Source: CAD feature listing. Evaluate the final solid. Frame: model axes, mm. Round coordinates to 2 decimals unless told otherwise and drop trailing zeros. Order: outer loops, then holes, each group sorted by start corner. A loop starts at its lowest first (then second) coordinate and runs counter-clockwise, first axis right, second up.
```python
from build123d import *

# Parameters (mm, degrees)
SKETCH1_R           = 29
BOSS_EXTRUDE1_DEPTH = 3
CUT_EXTRUDE1_DEPTH  = 3
SKETCH6_R           = 0.9
BOSS_EXTRUDE3_DEPTH = 2.5
SKETCH7_R           = 0.9
BOSS_EXTRUDE4_DEPTH = 2.5
SKETCH8_R           = 5
CUT_EXTRUDE2_DEPTH  = 3


with BuildPart() as part:
    # Sketch1 → Boss-Extrude1 (new body)
    with BuildSketch(Plane(origin=(0, 0, 0), x_dir=(1, 0, 0), z_dir=(0, 1, 0))):
        with Locations(Location((0, 0, 0), (0, 0, 270))):
            Circle(SKETCH1_R)
    extrude(amount=BOSS_EXTRUDE1_DEPTH)

    # Sketch2 → Cut-Extrude1 (cut)
    with BuildSketch(Plane(origin=(0, 3, 0), x_dir=(1, 0, 0), z_dir=(0, 1, 0))):
        Polygon((0, 29), (6.5, 29), (6.5, 18), (-6.5, 18), (-6.5, 29), align=None)
    extrude(amount=-CUT_EXTRUDE1_DEPTH, mode=Mode.SUBTRACT)

    # Sketch6 → Boss-Extrude3 (add)
    with BuildSketch(Plane(origin=(0, 3, 0), x_dir=(1, 0, 0), z_dir=(0, 1, 0))):
        with Locations(Location((-26, 0, 0), (0, 0, 270))):
            Circle(SKETCH6_R)
        with Locations(Location((26, 0, 0), (0, 0, 270))):
            Circle(SKETCH6_R)
    extrude(amount=BOSS_EXTRUDE3_DEPTH)

    # Sketch7 → Boss-Extrude4 (add)
    with BuildSketch(Plane(origin=(0, 3, 0), x_dir=(1, 0, 0), z_dir=(0, 1, 0))):
        with Locations(Location((0, -26, 0), (0, 0, 270))):
            Circle(SKETCH7_R)
    extrude(amount=BOSS_EXTRUDE4_DEPTH)

    # Sketch8 → Cut-Extrude2 (cut)
    with BuildSketch(Plane(origin=(0, 3, 0), x_dir=(1, 0, 0), z_dir=(0, 1, 0))):
        with Locations(Location((0, 0, 0), (0, 0, 270))):
            Circle(SKETCH8_R)
    extrude(amount=-CUT_EXTRUDE2_DEPTH, mode=Mode.SUBTRACT)


solid = part.part
```
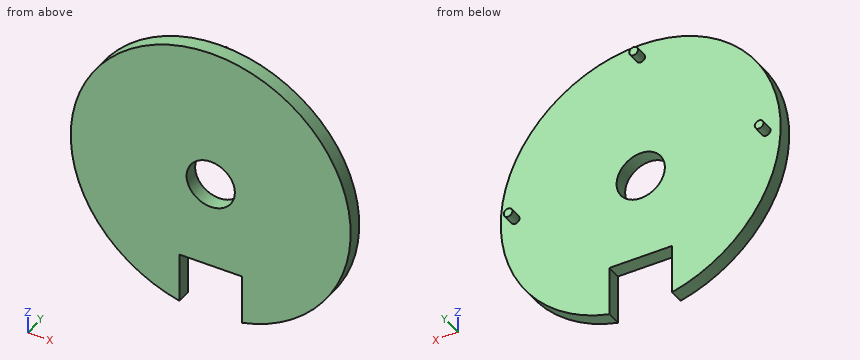
1. Section C-C on y = 1.1. Return loops of the section in (x, z).
2. Section D-D on x = -26. Return loops of the section in (y, z), plus the area to 3 significant figures.
3. Section A-A on x = 0. Return loops of the section in (y, z), plus the area to 4 significant figures.
4. Section B-B on z = 0. Return loops of the section in (x, y), plus the area to 3 significant figures.
5. First-contact query: pin 1 (1 mm diameter, centred on x = -20.5, y = 2.5, fed in from -Z); pin 2 (1.5 mm diameter, centred on x = -3, y = 1, fed in from -Z); pin 3 (4 mm diameter, centred on x = -22.5, z = -0.5, fed in from -Y); pin 4 (2 mm diameter, centred on y = 2, z = 1.5, fed in from -X). Flat tips, straight axial feed; report the tip coordinate or a pass-through.
6. Line query: line 1 along X through (y, z) = (1.1, 0); line 2 along Y through (x, z) = (13.5, -13); line 3 along Z through (x, y) = (-14.5, 1.45). Output: solid intervals per line, ascending.
Result:
1. outline: (-6.5, -28.26) - (-6.5, -18) - (6.5, -18) - (6.5, -28.26) arc R29 ccw (long way) to start; hole circle Ø10 at (0, 0)
2. outline: (0, -12.85) - (3, -12.85) - (3, -0.9) - (5.5, -0.9) - (5.5, 0.9) - (3, 0.9) - (3, 12.85) - (0, 12.85) - close
2. area: 81.6 mm2
3. outline: (0, -18) - (3, -18) - (3, -5) - (0, -5) - close; (0, 5) - (3, 5) - (3, 25.1) - (5.5, 25.1) - (5.5, 26.9) - (3, 26.9) - (3, 29) - (0, 29) - close
3. area: 115.5 mm2
4. outline: (-29, 0) - (-5, 0) - (-5, 3) - (-25.1, 3) - (-25.1, 5.5) - (-26.9, 5.5) - (-26.9, 3) - (-29, 3) - close; (5, 0) - (29, 0) - (29, 3) - (26.9, 3) - (26.9, 5.5) - (25.1, 5.5) - (25.1, 3) - (5, 3) - close
4. area: 153 mm2
5. pin 1: stops at z = -21
5. pin 2: stops at z = -18
5. pin 3: stops at y = 0
5. pin 4: stops at x = -29
6. line 1: x = -29 to -5, 5 to 29
6. line 2: y = 0 to 3
6. line 3: z = -25.11 to 25.11
